Check sheet for the modelled part. Datum: model origin and axes. Units: mm. Face numbers are marked on the shaded views. Round coordinates to 2 decimals unless told otherwise and drop trailing zeros. Write each loop counter-clockwise with the first axis right and the second up, starting at its lowest first coordinate (ties: lowest second). Pieces come first, ordered by that corner, then holes. Notation, with made-up numbers: (-20, 28.25) -> (32, 28.25) arc R32 cw to (32, 67.25) -> close; hole circle Ø8 at (-38.5, 25). An arc over 180 degrees is marked (long way). Use one line per item in the form item = value. Start each with the question number.
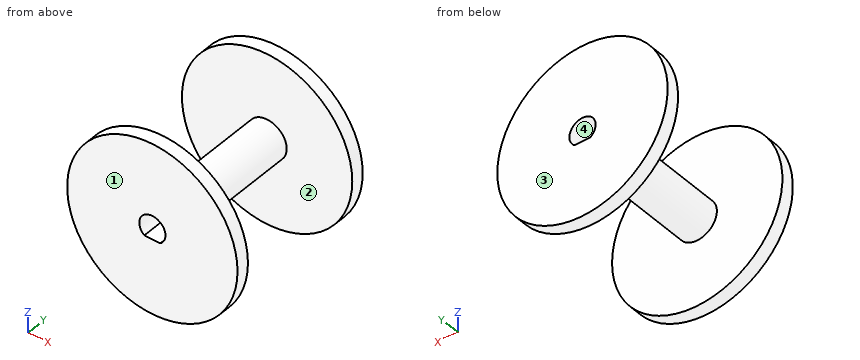
```python
from build123d import *

# Parameters (mm, degrees)
SKETCH1_R           = 33.02
BOSS_EXTRUDE1_DEPTH = 2.54
SKETCH2_R           = 3.81
SKETCH2_R_2         = 2.54
BOSS_EXTRUDE2_DEPTH = 25.4
SKETCH3_R           = 2.54
CUT_EXTRUDE1_DEPTH  = 25.4
SKETCH4_R           = 33.02
BOSS_EXTRUDE3_DEPTH = 2.54
SKETCH5_R           = 2.54
CUT_EXTRUDE2_DEPTH  = 2.54
BOSS_EXTRUDE4_DEPTH = 30.48
SKETCH7_R           = 33.02
SKETCH7_R_2         = 16.51
CUT_EXTRUDE3_DEPTH  = 132.842


with BuildPart() as part:
    # Sketch1 → Boss-Extrude1 (new body)
    with BuildSketch(Plane(origin=(0, 0, 0), x_dir=(1, 0, 0), z_dir=(0, 1, 0))):
        Circle(SKETCH1_R)
    extrude(amount=BOSS_EXTRUDE1_DEPTH)

    # Sketch2 → Boss-Extrude2 (add)
    with BuildSketch(Plane(origin=(0, 2.54, 0), x_dir=(1, 0, 0), z_dir=(0, 1, 0))):
        Circle(SKETCH2_R)
        Circle(SKETCH2_R_2, mode=Mode.SUBTRACT)
    extrude(amount=BOSS_EXTRUDE2_DEPTH)

    # Sketch3 → Cut-Extrude1 (cut)
    with BuildSketch(Plane(origin=(0, 2.54, 0), x_dir=(1, 0, 0), z_dir=(0, 1, 0))):
        Circle(SKETCH3_R)
    extrude(amount=-CUT_EXTRUDE1_DEPTH, mode=Mode.SUBTRACT)

    # Sketch4 → Boss-Extrude3 (add)
    with BuildSketch(Plane(origin=(0, 27.94, 0), x_dir=(1, 0, 0), z_dir=(0, 1, 0))):
        Circle(SKETCH4_R)
    extrude(amount=BOSS_EXTRUDE3_DEPTH)

    # Sketch5 → Cut-Extrude2 (cut)
    with BuildSketch(Plane.XZ.offset(-27.94)):
        Circle(SKETCH5_R)
    extrude(amount=-CUT_EXTRUDE2_DEPTH, mode=Mode.SUBTRACT)

    # Sketch6 → Boss-Extrude4 (add)
    with BuildSketch(Plane(origin=(0, 30.48, 0), x_dir=(1, 0, 0), z_dir=(0, 1, 0))):
        with BuildLine():
            Line((-1.557291379, 2.0066), (0, 2.0066))
            Line((0, 2.0066), (1.557291379, 2.0066))
            ThreePointArc((1.557291379, 2.0066), (0, 2.54), (-1.557291379, 2.0066))
        make_face()
    extrude(amount=-BOSS_EXTRUDE4_DEPTH)

    # Sketch7 → Cut-Extrude3 (cut)
    with BuildSketch(Plane(origin=(0, 30.48, 0), x_dir=(1, 0, 0), z_dir=(0, 1, 0))):
        Circle(SKETCH7_R)
        Circle(SKETCH7_R_2, mode=Mode.SUBTRACT)
    extrude(amount=-CUT_EXTRUDE3_DEPTH, mode=Mode.SUBTRACT)


solid = part.part
```
1. Sectioned sample at C-C (y = 19). Enter the section's corners in (x, z).
2. Depth check by flat-ended pin: pin 1 (8 mm diameter, centred on x = -11.5, y = 21.5, fed in from -Z); pin 2 (5 mm diameter, centred on x = 2, y = 24, fed in from -Z); pin 3 (1.5 mm diameter, centred on x = -3, y = 22.5, fed in from +Z); pin 4 (1.6 mm diameter, centred on x = 0.5, y = 18, fed in from +Z). Enter the tip coordinate at first touch or a pass-through.
3. Sectioned sample at A-A (z = 0). Enter the section's corners in (x, y), and give its area (3 significant figures).
4. Sectioned sample at D-D (z = -11.5). Enter the section's corners in (x, y).
5. Sectioned sample at B-B (x = 0). Enter the section's corners in (y, z), and give its area (3 significant figures).
6. Mould release check, pull along Y, two halves, no side actions. Record for the marked faces 1, 2, 3 and 4: +Y half, -Y half, draft (parallel to the pull), parting line (faces both ways), or undercut.
7. Scan lines: probe 1 along X at (y, z) = (23, 0); probe 2 along Y at (x, z) = (13.5, -0.5); probe 3 along Z at (x, y) = (1.5, 3). Record each from-to range of solid material in increasing order.
Returned:
q1.outline = circle Ø7.62 at (0, 0); hole (-1.56, -2.01) -> (1.56, -2.01) arc R2.54 ccw (long way) to start
q2.pin_1 = through
q2.pin_2 = -3.81
q2.pin_3 = 3.07
q2.pin_4 = 3.81
q3.outline = (-16.51, 0) -> (-2.54, 0) -> (-2.54, 30.48) -> (-16.51, 30.48) -> (-16.51, 27.94) -> (-3.81, 27.94) -> (-3.81, 2.54) -> (-16.51, 2.54) -> close; (2.54, 0) -> (16.51, 0) -> (16.51, 2.54) -> (3.81, 2.54) -> (3.81, 27.94) -> (16.51, 27.94) -> (16.51, 30.48) -> (2.54, 30.48) -> close
q3.area = 206 mm^2
q4.outline = (-11.85, 0) -> (11.85, 0) -> (11.85, 2.54) -> (-11.85, 2.54) -> close; (-11.85, 27.94) -> (11.85, 27.94) -> (11.85, 30.48) -> (-11.85, 30.48) -> close
q5.outline = (0, -16.51) -> (2.54, -16.51) -> (2.54, -3.81) -> (27.94, -3.81) -> (27.94, -16.51) -> (30.48, -16.51) -> (30.48, -2.01) -> (0, -2.01) -> close; (0, 2.54) -> (30.48, 2.54) -> (30.48, 16.51) -> (27.94, 16.51) -> (27.94, 3.81) -> (2.54, 3.81) -> (2.54, 16.51) -> (0, 16.51) -> close
q5.area = 223 mm^2
q6.face_1 = -Y half
q6.face_2 = undercut
q6.face_3 = +Y half
q6.face_4 = draft
q7.probe_1 = -3.81 to -2.54, 2.54 to 3.81
q7.probe_2 = 0 to 2.54, 27.94 to 30.48
q7.probe_3 = -3.5 to -2.01, 2.05 to 3.5
